Print and shaded views of the part. All mm, measured from the part's lowest x, y and z. A direction names the side the tool comes from. Round coordinates to 2 decimals unless told otherwise and drop trailing zeros. Write each loop counter-clockwise with the first axis right and the second up, starting at its lowest first coordinate (ties: lowest second). Pieces come first, ordered by that corner, then holes.
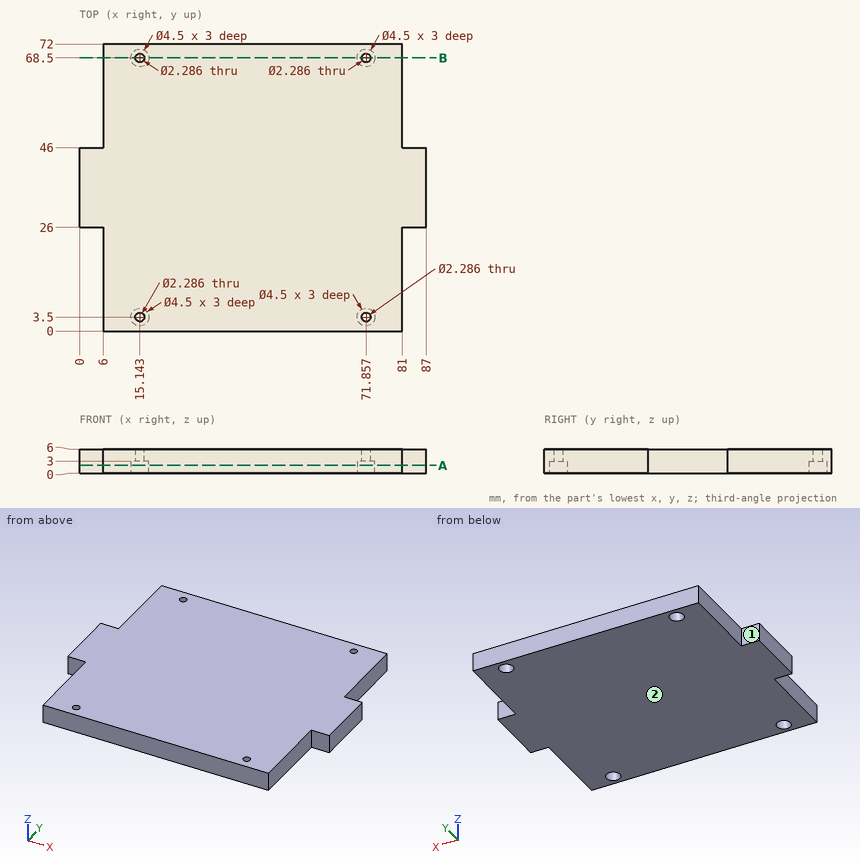
1) Slice it at A-A (z = 1.9). Write the cut outline in (x, y), plus the area to 3 significant figures.
Results:
outline: (0, 26) - (6, 26) - (6, 0) - (81, 0) - (81, 26) - (87, 26) - (87, 46) - (81, 46) - (81, 72) - (6, 72) - (6, 46) - (0, 46) - close; hole circle Ø4.5 at (15.14, 3.5); hole circle Ø4.5 at (15.14, 68.5); hole circle Ø4.5 at (71.86, 3.5); hole circle Ø4.5 at (71.86, 68.5)
area: 5,580 mm2
2) Wall check: L1, parallel to X at y = 3.5, z = 5.35; L2, parallel to X at y = 3.5, z = 0.85; L3, parallel to Y at x = 15, z = 2.8. Give the ranges that are in metal, low to high.
Results:
L1: x = 6 to 14, 16.29 to 70.71, 73 to 81
L2: x = 6 to 12.89, 17.39 to 69.61, 74.11 to 81
L3: y = 0 to 1.25, 5.75 to 66.25, 70.75 to 72
3) Pin check, flat tips, straight feed: pin 1 Ø2.5 at (x, y) = (15.143, 3.5) entering from -Z; pin 2 Ø4 at (x, y) = (15.143, 3.5) entering from +Z; pin 3 Ø3 at (y, z) = (9, 2.5) entering from -X. Stop position of each tip, or through.
Results:
pin 1: stops at z = 3
pin 2: stops at z = 6
pin 3: stops at x = 6
4) Which spindle directions (+Z, -Z, +X, -X, +Y, -Y) get a long thin tool onto all of the face, cutting with end or side? Do the marked faces 1 and 2. Say none if no direction does.
Results:
face 1: +Z, -Z, -X, +Y
face 2: -Z, +X, -X, +Y, -Y
5) Slice it at B-B (y = 68.5). Write the cut outline in (x, z), plus the area to 3 significant figures.
Results:
outline: (6, 0) - (12.89, 0) - (12.89, 3) - (14, 3) - (14, 6) - (6, 6) - close; (16.29, 3) - (17.39, 3) - (17.39, 0) - (69.61, 0) - (69.61, 3) - (70.71, 3) - (70.71, 6) - (16.29, 6) - close; (73, 3) - (74.11, 3) - (74.11, 0) - (81, 0) - (81, 6) - (73, 6) - close
area: 409 mm2
